Answer from the drawing. Dimensions are ordinates in mm from the lowest x, y and z of the part. Coordinates: 2 decimals unless noted, no trailing zeros. Order: outer loops, then holes, each group sorted by start corner. A loop starts at its lowest first (then second) coordinate and runs counter-clockwise, first axis right, second up. Notation, with made-up numbers: (39.5, 56.25) - (63.5, 56.25) arc R15 ccw to (63.5, 79.25) - close; hole circle Ø4 at (36.25, -11). An arc over 180 degrees is marked (long way). Answer as a JSON object with one key per item and string values. Group by question number.
1) Section A-A (z = 7) is taken. Give the vertices of the cut face in (x, y).
2) Find the intervals of material crossed by line 1 along Y through (x, z) = (67.5, 15.5) (1 decimal); line 2 along Y through (x, z) = (31.5, 12) (1 decimal); line 3 along X through (y, z) = (39, 19.5) (1 decimal), in increasing order.
3) Each of these flat-tipped pins is pushed along its axis until it touches: P1, Ø10, axis at y = 9, z = 22.5, coming from the +X side; P2, Ø2, axis at y = 59, z = 12, coming from the -X side; P3, Ø4, axis at x = 21.5, z = 13, coming from the -Y side. Where does it stop, or does it pass through?
4) The mould has two halves that part along Y. Classify the marked faces 1, 2 and 3: released by +Y, released by -Y, zero draft, split by the parting line, or undercut.
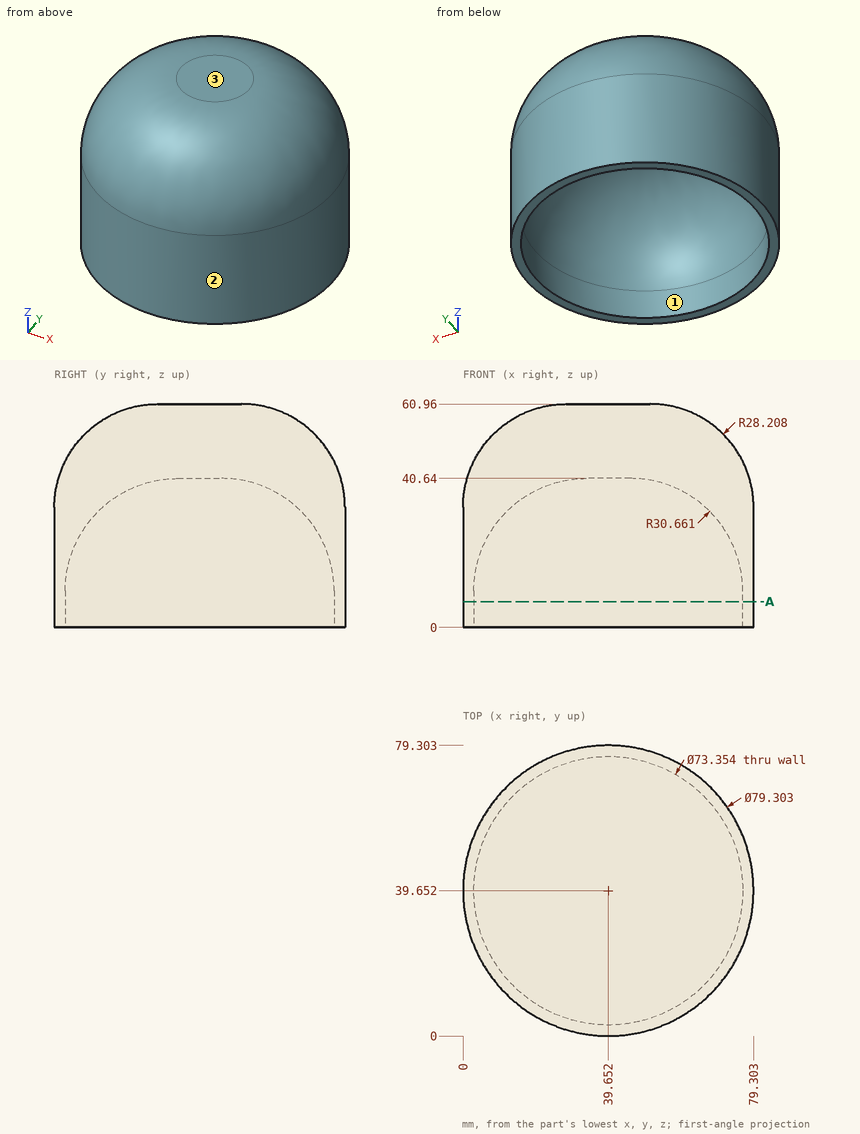
Report:
{
 "1": {"outline": "circle Ø79.3 at (39.65, 39.65); hole circle Ø73.35 at (39.65, 39.65)"},
 "2": {"line 1": "y = 11.4 to 16.6, 62.7 to 67.9", "line 2": "y = 0.8 to 4, 75.3 to 78.5", "line 3": "x = 0 to 4.5, 74.8 to 79.3"},
 "3": {"P1": "stops at x = 69.89", "P2": "stops at x = 4.5", "P3": "stops at y = 3.44"},
 "4": {"face 1": "undercut", "face 2": "split by the parting line", "face 3": "zero draft"}
}
